The listing builds one solid part. Answer for the finished solid, in the listing's coordinates (mm). Face numbers are marked on the shaded views. A direction names the side the tool comes from. Coordinates: 2 decimals unless noted, no trailing zeros. Order: outer loops, then holes, each group sorted by start corner. A loop starts at its lowest first (then second) coordinate and runs counter-clockwise, first axis right, second up.
```python
from build123d import *

# Parameters (mm, degrees)
F1_DEPTH = 25.4
F3_DEPTH = 152.4
F4_R     = 17.976868
F5_DEPTH = 177.801


with BuildPart() as f1:
    # F0 (on Front) → F1 (new body)
    with BuildSketch(Plane.XZ):
        Polygon((-177.8, 0), (0, 0), (-88.9, 165.1), (-177.8, 165.1), align=None)
    extrude(amount=F1_DEPTH)

    # F2 (on face) → F3 (join)
    with BuildSketch(Plane.XZ.offset(25.4)):
        Polygon((-177.8, 140.421584), (-177.8, 0), (-20.454695, 0), (-101.619244, 140.421584), align=None)
    extrude(amount=F3_DEPTH)

    # F4 (on face) → F5 (cut, through all)
    with BuildSketch(Plane(origin=(-177.8, 0, 0), x_dir=(0, -1, 0), z_dir=(-1, 0, 0))):
        with Locations((101.6, 70.880428)):
            Circle(F4_R)
    extrude(amount=-F5_DEPTH, mode=Mode.SUBTRACT)


solid = f1.part
```
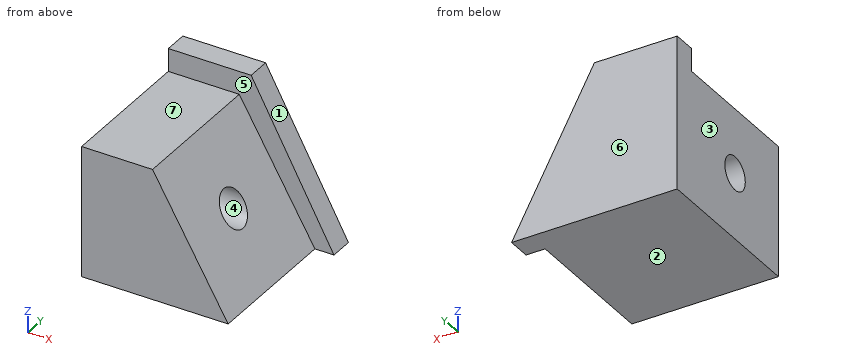
(1) Find section B-B (x = -133.5). Write down the section's boundary in (y, z).
(2) Consider line 1 (Z direction, x = -140, y = -101.6); line 2 (Y direction, x = -64.5, z = 85.5); line 3 (Z direction, x = -78, y = -92.5). Determine where each line is inside the solid, lowest interval first.
(3) The mould has two halves that part along Z. Classify the marked faces 1, 2, 3 and 4: released by +Z, released by -Z, zero draft, split by the parting line, or undercut.
(4) Find section A-A (z = 58). Write down the section's boundary in (x, y).
(5) Find section D-D (x = -59). Write down the section's boundary in (y, z).
(6) Each of these flat-tipped pins is pushed along its axis until it touches: pin 1 Ø5 at (y, z) = (-20, 32) entering from +X; pin 2 Ø2 at (x, y) = (-160, -153) entering from +Z; pin 3 Ø8 at (y, z) = (-115.5, 41.5) entering from +X. Where does it stop, or does it pass through?
(7) Find section C-C (y = -101.6). Write down the section's boundary in (x, z), and give its area (3 significant figures).
(8) For the marked faces 5, 6 and 7, determine the directions among +Z, -Z, +X, -X, +Y, -Y from which every point of the face is accessible in a straight line to the end or side of a thin tool.
Findings below:
1. outline: (-177.8, 0) - (0, 0) - (0, 165.1) - (-25.4, 165.1) - (-25.4, 140.42) - (-177.8, 140.42) - close; hole circle Ø35.95 at (-101.6, 70.88)
2. line 1: z = 0 to 52.9, 88.86 to 140.42
2. line 2: y = -25.4 to 0
2. line 3: z = 0 to 55.38, 86.38 to 99.56
3. face 1: released by +Z
3. face 2: released by -Z
3. face 3: zero draft
3. face 4: undercut
4. outline: (-177.8, -177.8) - (-53.98, -177.8) - (-53.98, -114.14) - (-177.8, -114.14) - close; (-177.8, -89.06) - (-53.98, -89.06) - (-53.98, -25.4) - (-31.23, -25.4) - (-31.23, 0) - (-177.8, 0) - close
5. outline: (-177.8, 0) - (0, 0) - (0, 109.57) - (-25.4, 109.57) - (-25.4, 66.69) - (-84.12, 66.69) arc R17.98 cw to (-119.08, 66.69) - (-177.8, 66.69) - close
6. pin 1: stops at x = -15.88
6. pin 2: stops at z = 140.42
6. pin 3: stops at x = -42.13
7. outline: (-177.8, 0) - (-20.45, 0) - (-51.03, 52.9) - (-177.8, 52.9) - close; (-177.8, 88.86) - (-71.81, 88.86) - (-101.62, 140.42) - (-177.8, 140.42) - close
7. area: 12,200 mm2
8. face 5: +Z, +X, -Y
8. face 6: +Z, -Z, +X, -X, +Y
8. face 7: +Z, +X, -X, -Y
